```python
from build123d import *

# Parameters (mm, degrees)
F0_R     = 3.175
F1_DEPTH = 25.4


with BuildPart() as f1:
    # F0 (on Front) → F1 (new body)
    with BuildSketch(Plane.XZ):
        with BuildLine():
            ThreePointArc((-9.525, 0), (0, -9.525), (9.525, 0))
            ThreePointArc((9.525, 0), (0, 9.525), (-9.525, 0))
        make_face()
        Circle(F0_R, mode=Mode.SUBTRACT)
        with BuildLine():
            Line((15.747457, -48.791711), (9.525, 0))
            ThreePointArc((9.525, 0), (0, -9.525), (-9.525, 0))
            Line((-9.525, 0), (-15.747457, -48.791711))
            ThreePointArc((-15.747457, -48.791711), (0, -34.925), (15.747457, -48.791711))
        make_face()
        with Locations((-3.175, -14.2748)):
            Circle(F0_R, mode=Mode.SUBTRACT)
        with BuildLine():
            ThreePointArc((15.875, -50.8), (15.843082, -49.793832), (15.747457, -48.791711))
            ThreePointArc((15.747457, -48.791711), (0, -34.925), (-15.747457, -48.791711))
            ThreePointArc((-15.747457, -48.791711), (-15.873588, -50.588243), (-15.795426, -52.3875))
            ThreePointArc((-15.795426, -52.3875), (0, -66.675), (15.795426, -52.3875))
            ThreePointArc((15.795426, -52.3875), (15.855094, -51.594747), (15.875, -50.8))
        make_face()
        with Locations((0, -50.8)):
            Circle(F0_R, mode=Mode.SUBTRACT)
        with BuildLine():
            ThreePointArc((15.795426, -52.3875), (0, -66.675), (-15.795426, -52.3875))
            Line((-15.795426, -52.3875), (-9.477255, -115.2525))
            ThreePointArc((-9.477255, -115.2525), (-0.476848, -104.786944), (9.525, -114.3))
            ThreePointArc((9.525, -114.3), (6.970557, -120.791299), (0.677344, -123.800886))
            Line((0.677344, -123.800886), (44.732405, -122.232475))
            ThreePointArc((44.732405, -122.232475), (36.512523, -114.280693), (44.770992, -106.368993))
            Line((44.770992, -106.368993), (18.942263, -105.323627))
            ThreePointArc((18.942263, -105.323627), (13.261089, -102.592755), (11.353419, -96.584911))
            Line((11.353419, -96.584911), (15.795426, -52.3875))
        make_face()
        with BuildLine():
            ThreePointArc((9.525, -114.3), (-0.476848, -104.786944), (-9.477255, -115.2525))
            ThreePointArc((-9.477255, -115.2525), (-6.389564, -121.363929), (0, -123.825))
            Line((0, -123.825), (0.677344, -123.800886))
            ThreePointArc((0.677344, -123.800886), (6.970557, -120.791299), (9.525, -114.3))
        make_face()
        with Locations((0, -114.3)):
            Circle(F0_R, mode=Mode.SUBTRACT)
        with BuildLine():
            Line((0.677344, -123.800886), (0, -123.825))
            ThreePointArc((0, -123.825), (0.338886, -123.81897), (0.677344, -123.800886))
        make_face()
        with BuildLine():
            ThreePointArc((52.3875, -114.3), (50.175023, -108.801999), (44.770992, -106.368993))
            ThreePointArc((44.770992, -106.368993), (36.512523, -114.280693), (44.732405, -122.232475))
            ThreePointArc((44.732405, -122.232475), (50.161633, -119.81191), (52.3875, -114.3))
        make_face()
        with Locations((44.45, -114.3)):
            Circle(F0_R, mode=Mode.SUBTRACT)
    extrude(amount=F1_DEPTH)


solid = f1.part
```
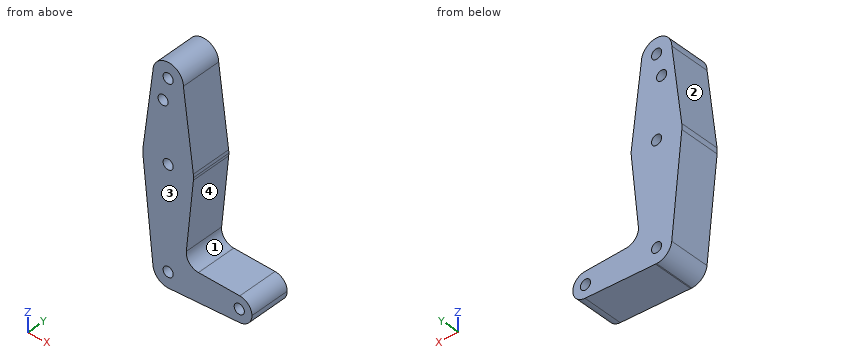
Here's how the part is built. I have some questions about the finished solid (model axes, mm). Face numbers are marked on the shaded views. Coordinates: 2 decimals unless noted, no trailing zeros. Loops run counter-clockwise (first coordinate to the right, second up) from the corner with the lowest first, then second, coordinate; pieces in that order, holes last. Notation, with made-up numbers: (86, -38) - (108, -38) arc R15 cw to (108, -16) - close; hole circle Ø3 at (-22, -17.5). An arc over 180 degrees is marked (long way). Return JSON: item names as keys, results as strings. Group by question number.
Item 1: If we section it at B-B on x = 37: Write out the boundary of the cut face in (y, z).
Item 2: If we section it at C-C on z = -82.5: Write out the boundary of the cut face in (x, y).
Item 3: Will these pins go through, and if not, where does the flat tip stop? P1, Ø1.5, axis at y = -14.5, z = -37, coming from the +X side; P2, Ø8, axis at y = -6.5, z = -52.5, coming from the +X side (3 decimals); P3, Ø5, axis at x = 19.5, y = -19, coming from the +Z side.
Item 4: If we section it at A-A on y = -20.5: State how many separate pieces and enclosed holes the cut face has, and give its area (3 significant figures).
Item 5: We'd pull the mould along Z, two halves only. Please class the marked faces 1, 2, 3 and 4: +Z half, -Z half, draft (parallel to the pull), parting line (faces both ways), or undercut.
Item 6: I need wall thicknesses on line 1 (Z direction, x = 44.45, y = -19) (3 decimals); line 2 (Z direction, x = 45.5, y = -2.5); line 3 (X direction, y = -17.5, z = -10). Which ranges of each line are inside material? Lowest first, please. Write a range as from..to.
Calculated:
{
 "1": {"outline": "(-25.4, -122.51) - (0, -122.51) - (0, -106.05) - (-25.4, -106.05) - close"},
 "2": {"outline": "(-12.77, -25.4) - (12.77, -25.4) - (12.77, 0) - (-12.77, 0) - close"},
 "3": {"P1": "stops at x = 14.34", "P2": "stops at x = 15.875", "P3": "stops at z = -105"},
 "4": {"separate pieces": "1", "enclosed holes": "5", "area": "3,770 mm^2"},
 "5": {"face 1": "undercut", "face 2": "+Z half", "face 3": "draft", "face 4": "undercut"},
 "6": {"line 1": "z = -122.243..-117.475, -111.125..-106.356", "line 2": "z = -122.17..-117.3, -111.3..-106.43", "line 3": "x = -10.8..10.8"}
}
